Geometry check sheet. Reference: the model listing, model coordinates, mm. A direction names the side the tool comes from. Round coordinates to 2 decimals unless told otherwise and drop trailing zeros. Loops run counter-clockwise (first coordinate to the right, second up) from the corner with the lowest first, then second, coordinate; pieces in that order, holes last. Notation, with made-up numbers: M -28.75,38 L 13.25,38 A12 cw 13.25,59 Z; hole C 56,2.5 d11. An arc over 180 degrees is marked long. Write item = value, one per line.
from build123d import *

# Parameters (mm, degrees)
SKETCH_1_W           = 89
SKETCH_1_H           = 37.5
EXTRUDE_1_DEPTH      = 8.5
SKETCH_2_W           = 85
SKETCH_2_H           = 33.5
CUT_EXTRUDE_1_DEPTH  = 7
CUT_EXTRUDE_3_DEPTH  = 4
FILLET_1_R           = 2
EXTRUDE_2_DEPTH      = 1
SKETCH_10_R          = 2.5
EXTRUDE_3_DEPTH      = 4.5
SKETCH_11_R          = 0.79
CUT_EXTRUDE_9_DEPTH  = 3
SKETCH_8_R           = 7.5
CUT_EXTRUDE_8_DEPTH  = 3
SKETCH_7_R           = 10
CUT_EXTRUDE_7_DEPTH  = 3
CUT_EXTRUDE_START    = -2.5
CUT_EXTRUDE_10_DEPTH = 2.5
CUT_EXTRUDE_11_DEPTH = 10


with BuildPart() as part:
    # 草图1 → 凸台-拉伸1 (new body)
    with BuildSketch(Plane.XY):
        Rectangle(SKETCH_1_W, SKETCH_1_H)
    extrude(amount=EXTRUDE_1_DEPTH)

    # 草图2 → 切除-拉伸1 (cut)
    with BuildSketch(Plane(origin=(0, 0, 0), x_dir=(-1, 0, 0), z_dir=(0, 0, -1))):
        Rectangle(SKETCH_2_W, SKETCH_2_H)
    extrude(amount=-CUT_EXTRUDE_1_DEPTH, mode=Mode.SUBTRACT)

    # 草图3 → 切除-拉伸3 (cut)
    with BuildSketch(Plane(origin=(44.5, 0, 0), x_dir=(0, 0, -1), z_dir=(1, 0, 0))):
        with BuildLine():
            Line((0, 1.6), (0, -1.6))
            Line((0, -1.6), (-1.5, -1.6))
            ThreePointArc((-1.5, -1.6), (-3.1, 0), (-1.5, 1.6))
            Line((-1.5, 1.6), (0, 1.6))
        make_face()
    extrude(amount=-CUT_EXTRUDE_3_DEPTH, mode=Mode.SUBTRACT)

    # 圆角1
    fillet_1_edges = [part.edges().sort_by_distance(p)[0] for p in [
        (-44.5, 0, 8.5),
        (0, -18.75, 8.5),
        (42.5, -16.75, 3.5),
        (42.5, 16.75, 3.5),
        (-42.5, 16.75, 3.5),
        (-42.5, -16.75, 3.5),
        (44.5, 0, 8.5),
        (0, 18.75, 8.5),
        (44.5, -18.75, 4.25),
        (-44.5, -18.75, 4.25),
        (-44.5, 18.75, 4.25),
        (44.5, 18.75, 4.25),
    ]]
    fillet(fillet_1_edges, radius=FILLET_1_R)

    # 草图9 → 凸台-拉伸2 (add)
    with BuildSketch(Plane(origin=(0, 0, 0), x_dir=(-1, 0, 0), z_dir=(0, 0, -1))):
        with BuildLine():
            Line((-43.5, 15.75), (-43.5, 1.6))
            Line((-43.5, 1.6), (-42.5, 1.6))
            Line((-42.5, 1.6), (-42.5, 14.75))
            ThreePointArc((-42.5, 14.75), (-41.914213562, 16.164213562), (-40.5, 16.75))
            Line((-40.5, 16.75), (40.5, 16.75))
            ThreePointArc((40.5, 16.75), (41.914213562, 16.164213562), (42.5, 14.75))
            Line((42.5, 14.75), (42.5, -14.75))
            ThreePointArc((42.5, -14.75), (41.914213562, -16.164213562), (40.5, -16.75))
            Line((40.5, -16.75), (-40.5, -16.75))
            ThreePointArc((-40.5, -16.75), (-41.914213562, -16.164213562), (-42.5, -14.75))
            Line((-42.5, -14.75), (-42.5, -1.6))
            Line((-42.5, -1.6), (-43.5, -1.6))
            Line((-43.5, -1.6), (-43.5, -15.75))
            ThreePointArc((-43.5, -15.75), (-42.914213562, -17.164213562), (-41.5, -17.75))
            Line((-41.5, -17.75), (41.5, -17.75))
            ThreePointArc((41.5, -17.75), (42.914213562, -17.164213562), (43.5, -15.75))
            Line((43.5, -15.75), (43.5, 15.75))
            ThreePointArc((43.5, 15.75), (42.914213562, 17.164213562), (41.5, 17.75))
            Line((41.5, 17.75), (-41.5, 17.75))
            ThreePointArc((-41.5, 17.75), (-42.914213562, 17.164213562), (-43.5, 15.75))
        make_face()
    extrude(amount=EXTRUDE_2_DEPTH)

    # 草图10 → 凸台-拉伸3 (add)
    with BuildSketch(Plane(origin=(0, 0, 7), x_dir=(-1, 0, 0), z_dir=(0, 0, -1))):
        with Locations((39.3, -13.35)):
            Circle(SKETCH_10_R)
        with Locations((39.3, 13.35)):
            Circle(SKETCH_10_R)
        with Locations((-34.5, 13.35)):
            Circle(SKETCH_10_R)
        with Locations((-34.5, -13.35)):
            Circle(SKETCH_10_R)
    extrude(amount=EXTRUDE_3_DEPTH)

    # 草图11 → 切除-拉伸9 (cut)
    with BuildSketch(Plane(origin=(0, 0, 2.5), x_dir=(-1, 0, 0), z_dir=(0, 0, -1))):
        with Locations((-34.5, 13.35)):
            Circle(SKETCH_11_R)
        with Locations((-34.5, -13.35)):
            Circle(SKETCH_11_R)
        with Locations((39.3, 13.35)):
            Circle(SKETCH_11_R)
        with Locations((39.3, -13.35)):
            Circle(SKETCH_11_R)
    extrude(amount=-CUT_EXTRUDE_9_DEPTH, mode=Mode.SUBTRACT)

    # 草图8 → 切除-拉伸8 (cut)
    with BuildSketch(Plane(origin=(0, 0, 7), x_dir=(-1, 0, 0), z_dir=(0, 0, -1))):
        with Locations((-1, -0.55)):
            Circle(SKETCH_8_R)
    extrude(amount=-CUT_EXTRUDE_8_DEPTH, mode=Mode.SUBTRACT)

    # 草图7 → 切除-拉伸7 (cut)
    with BuildSketch(Plane(origin=(0, 0, 7), x_dir=(-1, 0, 0), z_dir=(0, 0, -1))):
        with Locations((29.1, 0)):
            Circle(SKETCH_7_R)
    extrude(amount=-CUT_EXTRUDE_7_DEPTH, mode=Mode.SUBTRACT)

    # 草图13 → 切除-拉伸10 (cut)
    with BuildSketch(Plane(origin=(0, 0, -1), x_dir=(-1, 0, 0), z_dir=(0, 0, -1)).offset(CUT_EXTRUDE_START)):
        with BuildLine():
            Line((-41.5, 17.75), (41.5, 17.75))
            ThreePointArc((41.5, 17.75), (42.914213562, 17.164213562), (43.5, 15.75))
            Line((43.5, 15.75), (43.5, -15.75))
            ThreePointArc((43.5, -15.75), (42.914213562, -17.164213562), (41.5, -17.75))
            Line((41.5, -17.75), (-41.5, -17.75))
            ThreePointArc((-41.5, -17.75), (-42.914213562, -17.164213562), (-43.5, -15.75))
            Line((-43.5, -15.75), (-43.5, 15.75))
            ThreePointArc((-43.5, 15.75), (-42.914213562, 17.164213562), (-41.5, 17.75))
        make_face()
    extrude(amount=CUT_EXTRUDE_10_DEPTH, mode=Mode.SUBTRACT)

    # 草图14 → 切除-拉伸11 (cut)
    with BuildSketch(Plane(origin=(0, 0, 7), x_dir=(-1, 0, 0), z_dir=(0, 0, -1))):
        with BuildLine():
            Line((-21, -6.25), (-16, -6.25))
            ThreePointArc((-16, -6.25), (-15.646446609, -6.396446609), (-15.5, -6.75))
            Line((-15.5, -6.75), (-15.5, -9.75))
            ThreePointArc((-15.5, -9.75), (-15.646446609, -10.103553391), (-16, -10.25))
            Line((-16, -10.25), (-21, -10.25))
            ThreePointArc((-21, -10.25), (-21.353553391, -10.103553391), (-21.5, -9.75))
            Line((-21.5, -9.75), (-21.5, -6.75))
            ThreePointArc((-21.5, -6.75), (-21.353553391, -6.396446609), (-21, -6.25))
        make_face()
        with BuildLine():
            Line((-21, 10.25), (-16, 10.25))
            ThreePointArc((-16, 10.25), (-15.646446609, 10.103553391), (-15.5, 9.75))
            Line((-15.5, 9.75), (-15.5, 6.75))
            ThreePointArc((-15.5, 6.75), (-15.646446609, 6.396446609), (-16, 6.25))
            Line((-16, 6.25), (-21, 6.25))
            ThreePointArc((-21, 6.25), (-21.353553391, 6.396446609), (-21.5, 6.75))
            Line((-21.5, 6.75), (-21.5, 9.75))
            ThreePointArc((-21.5, 9.75), (-21.353553391, 10.103553391), (-21, 10.25))
        make_face()
    extrude(amount=-CUT_EXTRUDE_11_DEPTH, mode=Mode.SUBTRACT)


solid = part.part
(1) Release check for a two-part mould opening along X. For faces 1 (the cylindrical face through (0.59, 18.18, 7.9)), 2 (the cylindrical face through (43.9, -18.18, 3.3)), 3 (the cylindrical face through (-5.93, -3.42, 7.74)) record: released by +X, released by -X, zero draft, split by the parting line, or undercut.
Result set:
face_1 = zero draft
face_2 = released by +X
face_3 = undercut
(2) Tool access check on faces 4 (the flat face through (9, 0, 8.5)), 5 (the flat face through (-42.5, 0, 4)), 6 (the flat face through (15.5, 8, 8)). Record the directions out of +Z, -Z, +X, -X, +Y, -Y that give a thin tool (end or side, any length) a straight path to the whole face; none if there is none.
Result set:
face_4 = +Z, +X, -X, +Y, -Y
face_5 = -Z
face_6 = +Z, -Z
(3) Depth check by flat-ended pin: pin 1 Ø1.4 at (x, y) = (-39.3, -13.35) entering from -Z; pin 2 Ø0.8 at (y, z) = (-7.5, 7.5) entering from +X; pin 3 Ø0.8 at (y, z) = (7.5, 8) entering from -X. Enter the tip coordinate at first touch or a pass-through.
Result set:
pin_1 = 5.5
pin_2 = 44.41
pin_3 = -44.17
(4) Sectioned sample at B-B on x = 19. Record the cut outline in (y, z), then the cut area to 3 significant figures.
Result set:
outline = M -18.75,0 L -17.75,0 L -17.75,1.5 L -16.75,1.5 L -16.75,7 L -10.25,7 L -10.25,8.5 L -16.75,8.5 A2 ccw -18.75,6.5 Z; M -6.25,7 L 6.25,7 L 6.25,8.5 L -6.25,8.5 Z; M 10.25,7 L 16.75,7 L 16.75,1.5 L 17.75,1.5 L 17.75,0 L 18.75,0 L 18.75,6.5 A2 ccw 16.75,8.5 L 10.25,8.5 Z
area = 67.5 mm2
(5) Sectioned sample at D-D on x = 1. Record the cut outline in (y, z).
Result set:
outline = M -18.75,0 L -17.75,0 L -17.75,1.5 L -16.75,1.5 L -16.75,7 L -8.05,7 L -8.05,8.5 L -16.75,8.5 A2 ccw -18.75,6.5 Z; M 6.95,7 L 16.75,7 L 16.75,1.5 L 17.75,1.5 L 17.75,0 L 18.75,0 L 18.75,6.5 A2 ccw 16.75,8.5 L 6.95,8.5 Z
(6) Material ranges on line 1 along Y through (x, z) = (-39.3, 4.9); line 2 along Y through (x, z) = (-27, 6); line 3 along X through (y, z) = (16, 0.75), recorded low to high. Write a range as from..to.
Result set:
line_1 = -18.75..-16.75, -15.85..-14.14, -12.56..-10.85, 10.85..12.56, 14.14..15.85, 16.75..18.75
line_2 = -18.75..-16.75, 16.75..18.75
line_3 = -44.5..-43.48, 43.48..44.5
(7) Sectioned sample at A-A on x = -29.1. Record the cut outline in (y, z).
Result set:
outline = M -18.75,0 L -17.75,0 L -17.75,1.5 L -16.75,1.5 L -16.75,7 L -10,7 L -10,8.5 L -16.75,8.5 A2 ccw -18.75,6.5 Z; M 10,7 L 16.75,7 L 16.75,1.5 L 17.75,1.5 L 17.75,0 L 18.75,0 L 18.75,6.5 A2 ccw 16.75,8.5 L 10,8.5 Z
